```python
from build123d import *

# Parameters (mm, degrees)
SKETCH1_R           = 8.5
SKETCH1_W           = 12
SKETCH1_H           = 4.5
SKETCH1_W_2         = 11
SKETCH1_H_2         = 2.35
BOSS_EXTRUDE2_DEPTH = 3


with BuildPart() as part:
    # Sketch1 → Boss-Extrude2 (new body)
    with BuildSketch(Plane.XY):
        with BuildLine():
            Line((-67.723514566, 14.691706599), (-67.723514566, -5.058293401))
            Line((-67.723514566, -5.058293401), (-62.723514566, -5.058293401))
            Line((-62.723514566, -5.058293401), (-62.723514566, -9.058293401))
            Line((-62.723514566, -9.058293401), (-23.723514566, -9.058293401))
            Line((-23.723514566, -9.058293401), (-23.723514566, -5.058293401))
            Line((-23.723514566, -5.058293401), (-18.723514566, -5.058293401))
            Line((-18.723514566, -5.058293401), (-18.723514566, 14.691706599))
            ThreePointArc((-18.723514566, 14.691706599), (-19.968310746, 17.696910419), (-22.973514566, 18.941706599))
            Line((-22.973514566, 18.941706599), (-63.473514566, 18.941706599))
            ThreePointArc((-63.473514566, 18.941706599), (-66.478718386, 17.696910419), (-67.723514566, 14.691706599))
        make_face()
        with Locations((-56.223514566, 8.441706599)):
            Circle(SKETCH1_R, mode=Mode.SUBTRACT)
        with Locations((-30.223514566, 8.441706599)):
            Circle(SKETCH1_R, mode=Mode.SUBTRACT)
        with Locations((-43.240297901, 0.09191466)):
            Rectangle(SKETCH1_W, SKETCH1_H, mode=Mode.SUBTRACT)
        with Locations((-42.84448226, 16.979921864)):
            Rectangle(SKETCH1_W_2, SKETCH1_H_2, mode=Mode.SUBTRACT)
    extrude(amount=BOSS_EXTRUDE2_DEPTH)


solid = part.part
```
Here's how the part is built. I have some questions about the finished solid (model axes, mm). A direction names the side the tool comes from. Round coordinates to 2 decimals unless told otherwise and drop trailing zeros. Write each loop counter-clockwise with the first axis right and the second up, starting at its lowest first coordinate (ties: lowest second). Pieces come first, ordered by that corner, then holes. Notation, with made-up numbers: M -21.5,-25.75 L 29.5,-25.75 A12 cw 29.5,-3.75 Z; hole C -34,65 d10. An arc over 180 degrees is marked long. Answer as CSV lines item,"result". Start each with the question number.
1. Suppose I cut it at A-A on x = -42. Write out the boundary of the cut face in (y, z).
2. I need wall thicknesses on probe 1 along Y at (x, z) = (-47.5, 1.15); probe 2 along X at (y, z) = (-2, 2.5); probe 3 along Y at (x, z) = (-49, 0.4). Which ranges of each line are inside material? Lowest first, please.
3. On a 3-axis mill with a long thin cutter (end or side, diameter ignored), from which of +Z, -Z, +X, -X, +Y, -Y can I reach the whole of each face in a straight line? I mean faces 1 (the flat face through (-65, -5.058, 1)), 2 (the flat face through (-48.344, 17, 1)), 3 (the flat face through (-44, 5, 0)). Say none if no direction works.
4. Suppose I cut it at B-B on y = -1.25. Write out the boundary of the cut face in (x, z), then the cut area to 3 significant figures.
5. Thinking about a two-plate mould opening in X: for faces 4 (the flat face through (-43, 18.942, 1)), 5 (the cylindrical face through (-64.715, 8.815, 1.479)), 6 (the flat face through (-37.344, 17, 1)), 7 (the cylindrical face through (-19.935, 17.664, 1.479)), which applies, released by +X, released by -X, zero draft, split by the parting line, or undercut?
6. Suppose I cut it at C-C on x = -28.5. Write out the boundary of the cut face in (y, z), then the cut area to 3 significant figures.
7. Suppose I cut it at D-D on z = 2.2. Write out the boundary of the cut face in (x, y).
8. I'm going to push flat-ended pins straight in: pin 1 Ø0.9 at (x, z) = (-66, 1) entering from -Y; pin 2 Ø0.9 at (y, z) = (-7, 1) entering from +X. Where does each tip first touch, or does it pass through?
Check result:
1,outline,"M -9.06,0 L -2.16,0 L -2.16,3 L -9.06,3 Z; M 2.34,0 L 15.8,0 L 15.8,3 L 2.34,3 Z; M 18.15,0 L 18.94,0 L 18.94,3 L 18.15,3 Z"
2,probe 1,"y = -9.06 to -2.16, 2.34 to 15.8, 18.15 to 18.94"
2,probe 2,"x = -67.72 to -49.24, -37.24 to -18.72"
2,probe 3,"y = -9.06 to -2.16, 2.34 to 3.96, 12.92 to 18.94"
3,face 1,"+Z, -Z, -X, -Y"
3,face 2,"+Z, -Z"
3,face 3,"-Z, +X, -X, +Y, -Y"
4,outline,"M -67.72,0 L -49.24,0 L -49.24,3 L -67.72,3 Z; M -37.24,0 L -18.72,0 L -18.72,3 L -37.24,3 Z"
4,area,"111 mm2"
5,face 4,"zero draft"
5,face 5,"undercut"
5,face 6,"undercut"
5,face 7,"released by +X"
6,outline,"M -9.06,0 L 0.12,0 L 0.12,3 L -9.06,3 Z; M 16.77,0 L 18.94,0 L 18.94,3 L 16.77,3 Z"
6,area,"34.1 mm2"
7,outline,"M -67.72,-5.06 L -62.72,-5.06 L -62.72,-9.06 L -23.72,-9.06 L -23.72,-5.06 L -18.72,-5.06 L -18.72,14.69 A4.25 ccw -22.97,18.94 L -63.47,18.94 A4.25 ccw -67.72,14.69 Z; hole C -56.22,8.44 d17; hole M -49.24,-2.16 L -37.24,-2.16 L -37.24,2.34 L -49.24,2.34 Z; hole M -48.34,15.8 L -37.34,15.8 L -37.34,18.15 L -48.34,18.15 Z; hole C -30.22,8.44 d17"
8,pin 1,"stops at y = -5.06"
8,pin 2,"stops at x = -23.72"
